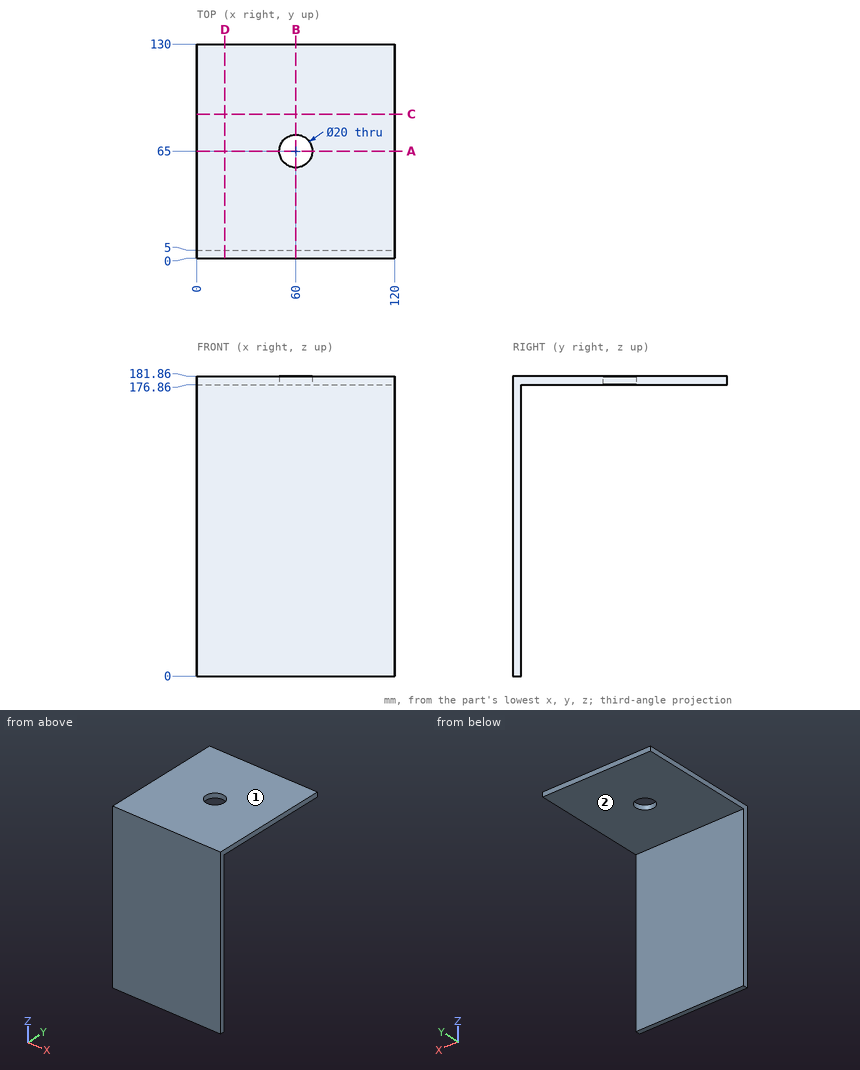
Geometry check sheet. Reference: drawing and pictorial views, mm from the part's lowest x, y, z. A direction names the side the tool comes from. Coordinates: 2 decimals unless noted, no trailing zeros. Order: outer loops, then holes, each group sorted by start corner. A loop starts at its lowest first (then second) coordinate and runs counter-clockwise, first axis right, second up. Notation, with made-up numbers: M 34.25,-26.75 L 78.25,-26.75 A32 ccw 78.25,11.25 Z; hole C 45.25,-0.5 d10. An arc over 180 degrees is marked long. Return JSON: item names as keys, results as strings.
1) Cross-section at D-D, the plane x = 17. Record the boundary of the cut face in (y, z).
Answer list:
{"outline": "M 0,0 L 5,0 L 5,176.86 L 130,176.86 L 130,181.86 L 0,181.86 Z"}
2) Gauge pin test, flat ends, axial feed: pin 1 (23 mm diameter, centred on x = 60, y = 65, fed in from -Z); pin 2 (12 mm diameter, centred on x = 76, z = 92.5, fed in from +Y); pin 3 (5 mm diameter, centred on x = 52.5, z = 111, fed in from -Y). Record the tip position at first contact, or that the pin passes through.
Answer list:
{"pin 1": "z = 176.86", "pin 2": "y = 5", "pin 3": "y = 0"}
3) Thickness scan on L1, parallel to Y at x = 60, z = 178; L2, parallel to X at y = 65, z = 180; L3, parallel to Y at x = 80, z = 43. Record the ranges inside material, lowest first. Write a range as [from, to].
Answer list:
{"L1": "[0, 55], [75, 130]", "L2": "[0, 50], [70, 120]", "L3": "[0, 5]"}
4) Cross-section at B-B, the plane x = 60. Record the boundary of the cut face in (y, z).
Answer list:
{"outline": "M 0,0 L 5,0 L 5,176.86 L 55,176.86 L 55,181.86 L 0,181.86 Z; M 75,176.86 L 130,176.86 L 130,181.86 L 75,181.86 Z"}
5) Cross-section at C-C, the plane y = 87.5. Record the boundary of the cut face in (x, z).
Answer list:
{"outline": "M 0,176.86 L 120,176.86 L 120,181.86 L 0,181.86 Z"}
6) Cross-section at A-A, the plane y = 65. Record the boundary of the cut face in (x, z).
Answer list:
{"outline": "M 0,176.86 L 50,176.86 L 50,181.86 L 0,181.86 Z; M 70,176.86 L 120,176.86 L 120,181.86 L 70,181.86 Z"}
7) Access from +Z, -Z, +X, -X, +Y, -Y to the whole of each face (thin tool, end or side, straight path). Record for the marked faces 1 and 2.
Answer list:
{"face 1": "+Z, +X, -X, +Y, -Y", "face 2": "-Z, +X, -X, +Y"}
